For this review, take the finished solid that the model builds, in its own axes (mm). Face numbers are marked on the shaded views. Round coordinates to 2 decimals unless told otherwise and drop trailing zeros. Write each loop counter-clockwise with the first axis right and the second up, starting at its lowest first coordinate (ties: lowest second). Pieces come first, ordered by that corner, then holes.
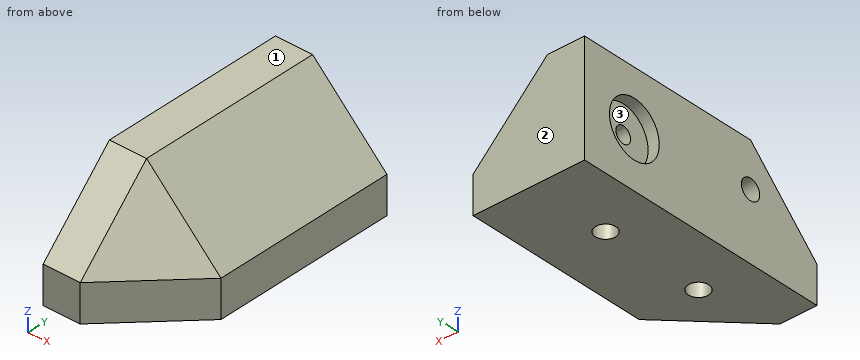
from build123d import *

# Parameters (mm, degrees)
SCHIZZO1_W                   = 30
SCHIZZO1_H                   = 40
ESTRUSIONE_ESTRUSIONE1_DEPTH = 30
SMUSSO1_SIZE                 = 20
ESTRUSIONE_ESTRUSIONE2_DEPTH = 30
FORO_PER_VITE_M5_1_D         = 5.5
FORO_PER_VITE_M5_1_DEPTH     = 13
FORO_PER_VITE_M5_1_TIP       = 1.652366702
FORO_PER_VITE_M5_2_D         = 5.5
FORO_PER_VITE_M5_2_DEPTH     = 13
FORO_PER_VITE_M5_2_TIP       = 1.652366702
SCHIZZO6_R                   = 7.5
TAGLIO_ESTRUSIONE1_DEPTH     = 3
FORO_PER_VITE_M4_1_D         = 4.4
FORO_PER_VITE_M4_1_DEPTH     = 10
FORO_PER_VITE_M4_1_TIP       = 1.321893362


with BuildPart() as part:
    # Schizzo1 → Estrusione-Estrusione1 (new body)
    with BuildSketch(Plane.XY):
        with Locations((15, 20)):
            Rectangle(SCHIZZO1_W, SCHIZZO1_H)
    extrude(amount=ESTRUSIONE_ESTRUSIONE1_DEPTH)

    # Smusso1
    smusso1_edges = [part.edges().sort_by_distance(p)[0] for p in [
        (30, 20, 30),
        (30, 0, 15),
        (15, 0, 30),
    ]]
    chamfer(smusso1_edges, length=SMUSSO1_SIZE)

    # Schizzo2 → Estrusione-Estrusione2 (add)
    with BuildSketch(Plane(origin=(0, 40, 0), x_dir=(1, 0, 0), z_dir=(0, 1, 0))):
        Polygon((0, 0), (30, 0), (30, -10), (10, -30), (0, -30), align=None)
    extrude(amount=ESTRUSIONE_ESTRUSIONE2_DEPTH)

    # Foro per Vite M5-1
    with Locations(Plane.ZY):
        with Locations((18, 20)):
            Hole(FORO_PER_VITE_M5_1_D / 2, depth=FORO_PER_VITE_M5_1_DEPTH)
            with Locations((0, 0, -(FORO_PER_VITE_M5_1_DEPTH + FORO_PER_VITE_M5_1_TIP / 2))):  # 118° drill point
                Cone(0, FORO_PER_VITE_M5_1_D / 2, FORO_PER_VITE_M5_1_TIP, mode=Mode.SUBTRACT)

    # Foro per Vite M5-2
    with Locations(Plane(origin=(14, 20, 0), x_dir=(-1, 0, 0), z_dir=(0, 0, -1))):
        with Locations((0, 0), (0, 28)):
            Hole(FORO_PER_VITE_M5_2_D / 2, depth=FORO_PER_VITE_M5_2_DEPTH)
            with Locations((0, 0, -(FORO_PER_VITE_M5_2_DEPTH + FORO_PER_VITE_M5_2_TIP / 2))):  # 118° drill point
                Cone(0, FORO_PER_VITE_M5_2_D / 2, FORO_PER_VITE_M5_2_TIP, mode=Mode.SUBTRACT)

    # Schizzo6 → Taglio-Estrusione1 (cut)
    with BuildSketch(Plane.ZY):
        with Locations((15, 55)):
            Circle(SCHIZZO6_R)
    extrude(amount=-TAGLIO_ESTRUSIONE1_DEPTH, mode=Mode.SUBTRACT)

    # Foro per Vite M4-1
    with Locations(Plane.ZY.offset(-3)):
        with Locations((15, 55)):
            Hole(FORO_PER_VITE_M4_1_D / 2, depth=FORO_PER_VITE_M4_1_DEPTH)
            with Locations((0, 0, -(FORO_PER_VITE_M4_1_DEPTH + FORO_PER_VITE_M4_1_TIP / 2))):  # 118° drill point
                Cone(0, FORO_PER_VITE_M4_1_D / 2, FORO_PER_VITE_M4_1_TIP, mode=Mode.SUBTRACT)


solid = part.part
(1) We need section B-B, the plane z = 4. Give the boundary of the cut face in (x, y).
Geometry check:
outline: (0, 0) - (10, 0) - (30, 20) - (30, 70) - (0, 70) - close; hole circle Ø5.5 at (14, 20); hole circle Ø5.5 at (14, 48)
(2) We need section C-C, the plane y = 6.5. Give the boundary of the cut face in (x, z).
Geometry check:
outline: (0, 0) - (16.5, 0) - (16.5, 10) - (10, 16.5) - (0, 16.5) - close
(3) Mouldability with a two-part tool opening along Z and no side actions: class the marked faces 1, 2 and 3 as pulls with the +Z half, pulls with the -Z half, needs draft (parallel to the pull), parting line crosses it, or undercut.
Geometry check:
face 1: pulls with the +Z half
face 2: needs draft
face 3: undercut
(4) For line 1 along X through (y, z) = (20, 5.25); line 2 along Y through (x, z) = (15, 13); line 3 along Y through (x, z) = (14, 4), list the stretches that pass through material, from the lowest coordinate up.
Geometry check:
line 1: x = 0 to 11.25, 16.75 to 30
line 2: y = 8 to 17.44, 22.56 to 45.44, 50.56 to 70
line 3: y = 4 to 17.25, 22.75 to 45.25, 50.75 to 70
(5) We need section D-D, the plane y = 64.5. Give the boundary of the cut face in (x, z), and give its area (3 significant figures).
Geometry check:
outline: (0, 0) - (30, 0) - (30, 10) - (10, 30) - (0, 30) - close
area: 700 mm2
(6) We need section A-A, the plane x = 8.5. Give the boundary of the cut face in (y, z).
Geometry check:
outline: (0, 0) - (70, 0) - (70, 30) - (20, 30) - (0, 10) - close; hole circle Ø5.5 at (20, 18); hole circle Ø4.4 at (55, 15)
(7) For pin 1 Ø3 at (y, z) = (17, 24.5) entering from +X; pin 2 Ø2.5 at (y, z) = (55, 15) entering from +X; pin 3 Ø5 at (x, y) = (14, 20) entering from -Z, all flat-tipped, find the tip position at first contact; note any pin that passes through.
Geometry check:
pin 1: stops at x = 14.62
pin 2: stops at x = 26.25
pin 3: stops at z = 13.15
